Autodesk Inventor part; units mm, degrees
ref_plane "YZ Plane" through (0, 0, 0) normal (1, 0, 0) x (0, 1, 0)
ref_plane "XZ Plane" through (0, 0, 0) normal (0, 1, 0) x (-1, 0, 0)
ref_plane "XY Plane" through (0, 0, 0) normal (0, 0, 1) x (1, 0, 0)
sketch "Sketch1" plane through (0, 0, 0) normal (0, 0, 1) x (1, 0, 0)
  circle A0 centre (0, 91.8009) radius 38.1 construction
  circle A1 centre (0, -91.8009) radius 38.1 construction
  line L0 (0, 91.8009) -> (0, -91.8009) construction
  circle A2 centre (-25.4, 0) radius 57.15 construction
  circle A3 centre (0, 91.8009) radius 14.2875
  circle A4 centre (0, -91.8009) radius 14.2875
  circle A5 centre (0, -91.8009) radius 33.3375 construction
  circle A6 centre (0, 91.8009) radius 33.3375 construction
  circle A7 centre (-142.9967, -39.6875) radius 14.3256 construction
  circle A8 centre (0, -91.8009) radius 23.876 construction
  line L1 (-142.9967, -39.6875) -> (0, -91.8009) construction
  circle A9 centre (-142.9967, 39.6875) radius 14.3256 construction
  circle A10 centre (0, 91.8009) radius 23.876 construction
  line L2 (0, 91.8009) -> (-142.9967, 39.6875) construction
  circle A11 centre (-142.9967, 39.6875) radius 39.6875 construction
  circle A12 centre (-142.9967, -39.6875) radius 39.6875 construction
  line L3 (-142.9967, 39.6875) -> (-142.9967, -39.6875) construction
  line L4 (-138.9458, 25.9466) -> (6.7516, 68.8994) construction
  line L5 (-9.5669, 113.6764) -> (-148.7368, 52.8128) construction
  line L6 (-138.9458, -25.9466) -> (6.7516, -68.8994) construction
  line L7 (-13.5443, -111.4635) -> (-134.8702, -27.89) construction
  circle A13 centre (-142.9967, 39.6875) radius 14.2875
  circle A14 centre (-142.9967, -39.6875) radius 14.2875
  circle A15 centre (-187.9418, -47.625) radius 5.9531 construction
  circle A16 centre (-187.9418, -47.625) radius 9.525
  circle A17 centre (-187.9418, -47.625) radius 17.4625 construction
  circle A18 centre (-187.9418, -47.625) radius 17.4625 construction
  circle A19 centre (-187.9418, -47.625) radius 17.4625 construction
  circle A20 centre (-187.9418, -47.625) radius 17.4625 construction
  circle A21 centre (-187.9418, -47.625) radius 17.4625 construction
  circle A22 centre (-19.05, 0) radius 57.15 construction
  circle A23 centre (-187.9418, -47.625) radius 26.9875
  line L8 (-241.3, 101.6) -> (-215.9, 101.6) construction
  line L9 (-215.9, 101.6) -> (-215.9, -101.6) construction
  line L10 (-215.9, -101.6) -> (-241.3, -101.6) construction
  line L11 (-241.3, -101.6) -> (-241.3, 101.6)
  line L12 (-142.9967, -39.6875) -> (-187.9418, -47.625) construction
  line L13 (-77.6563, 63.5) -> (-77.6563, -63.5) construction
  line L14 (-22.4906, -57.0463) -> (2.007, -58.5239)
  arc A24 (2.007, 58.5239) -> (27.142, 111.1581) centre (0, 91.8009) ccw
  arc A25 (-22.4906, 57.0463) -> (-22.4906, -57.0463) centre (-19.05, 0) ccw
  line L15 (2.007, 58.5239) -> (-22.4906, 57.0463)
  arc A26 (27.142, -111.1581) -> (2.007, -58.5239) centre (0, -91.8009) ccw
  arc A27 (3.8774, 143.7787) -> (-0.8591, 145.6978) centre (0, 141.0134) ccw
  circle A28 centre (0, 91.8009) radius 44.45 construction
  line L16 (3.8774, 143.7787) -> (27.142, 111.1581)
  line L17 (-0.8591, 145.6978) -> (-241.3, 101.6)
  arc A29 (-0.8591, -145.6978) -> (3.8774, -143.7787) centre (0, -141.0134) ccw
  line L18 (-241.3, -101.6) -> (-0.8591, -145.6978)
  line L19 (27.142, -111.1581) -> (3.8774, -143.7787)
  circle A30 centre (0, -91.8009) radius 44.45 construction
  line L20 (0, 112.8194) -> (0, 70.7824) construction
  line L21 (-142.9967, 60.706) -> (-142.9967, 18.669) construction
  line L22 (-142.9967, -18.669) -> (-142.9967, -60.706) construction
  line L23 (0, -70.7824) -> (0, -112.8194) construction
  line L24 (-228.6, 50.8) -> (-228.6, -50.8) construction
  line L25 (-187.9418, -15.875) -> (-187.9418, -79.375) construction
  circle A31 centre (-187.9418, -47.625) radius 17.4625 construction
  point P0 (0, 0)
  point P1 (0, 0)
  point P2 (-172.8189, -38.8937)
  point P3 (-187.9418, -30.1625)
  point P4 (-203.0648, -38.8938)
  point P5 (-203.0648, -56.3563)
  point P6 (-187.9418, -65.0875)
  point P7 (-215.9, 0)
  point P8 (-228.6, 0)
  point P9 (-228.6, 0)
  point P10 (-228.6, 101.6)
  point P11 (-172.8189, -56.3562)
  dimension "d15" = 34.925
  dimension "d0" = 76.2
  dimension "d1" = 76.2
  dimension "d2" = 114.3
  dimension "d4" = 183.6018
  dimension "d5" = 28.575
  dimension "d6" = 19.05
  dimension "d7" = 28.6512
  dimension "d8" = 47.752
  dimension "d9" = 79.375
  dimension "d10" = 142.9967
  dimension "d11" = 152.1968
  dimension "d12" = 28.575
  dimension "d13" = 11.9062
  dimension "d14" = 19.05
  dimension "d18" = 360
  dimension "d20" = 6.35
  dimension "d21" = 53.975
  dimension "d22" = 25.4
  dimension "d23" = 203.2
  dimension "d24" = 241.3
  dimension "d26" = 127
  dimension "d29" = 9.525
  dimension "d30" = 6.35
  dimension "d32" = 42.037
  dimension "d33" = 42.037
  dimension "d34" = 42.037
  dimension "d35" = 42.037
  dimension "d36" = 25.4
  dimension "d44" = 101.6
  dimension "d45" = 53.975
  dimension "d46" = 63.5
extrude "Extrusion1" add sketch "Sketch1" along normal blind 6.35 contours L11 L17 A27 L16 A24 L15 A25 L14 A26 L19 A29 L18
hole "Hole1" at (-172.8189, -38.8937, 0) at (-187.9418, -30.1625, 0) at (-203.0648, -38.8938, 0) at (-203.0648, -56.3563, 0) at (-187.9418, -65.0875, 0) at (-77.6563, 63.5, 0) at (-77.6563, -63.5, 0) at (0, 112.8194, 0) at (0, 70.7824, 0) at (-142.9967, 60.706, 0) at (-142.9967, 18.669, 0) at (-142.9967, -18.669, 0) at (-142.9967, -60.706, 0) at (0, -70.7824, 0) at (0, -112.8194, 0) at (-228.6, 50.8, 0) at (-228.6, 0, 0) at (-228.6, -50.8, 0) at (-187.9418, -79.375, 0) at (-187.9418, -15.875, 0) at (0, -141.0134, 0) at (0, 141.0134, 0) direction (0, 0, 1) diameter 5.1054 end through all
properties part number "GP6-002" material "Polycarbonate, Smoke"
Geometry: final body of the model. Coordinates: model frame, mm. A direction names the side the tool comes from. Give positions to 0.01 mm unless a question says otherwise; leave off trailing zeros. Write each loop counter-clockwise with the first axis right and the second up, starting at its lowest first coordinate (ties: lowest second). Pieces come first, ordered by that corner, then holes. Notation, with made-up numbers: (79, 7) -> (112, 7) arc R7 cw to (112, 15) -> close; hole circle Ø11 at (8, 6.5). An arc over 180 degrees is marked (long way). Answer in a Markdown table with one row per item.
(1) Section query A-A on x = -180. Return loops of the section in (y, z).
Answers below:
| item | result |
|---|---|
| outline | (-112.84, 0) -> (-73.42, 0) -> (-73.42, 6.35) -> (-112.84, 6.35) -> close; (-21.83, 0) -> (112.84, 0) -> (112.84, 6.35) -> (-21.83, 6.35) -> close |
(2) Section query B-B on z = 4. State how many separate pieces and enclosed holes the cut face has, then the cut area to 3 significant figures.
Answers below:
| item | result |
|---|---|
| separate pieces | 1 |
| enclosed holes | 22 |
| area | 51,200 mm^2 |
(3) Section query D-D on x = -19.05. Return loops of the section in (y, z), then the cut area to 3 significant figures.
Answers below:
| item | result |
|---|---|
| outline | (-142.36, 0) -> (-57.25, 0) -> (-57.25, 6.35) -> (-142.36, 6.35) -> close; (57.25, 0) -> (142.36, 0) -> (142.36, 6.35) -> (57.25, 6.35) -> close |
| area | 1,080 mm^2 |
(4) Ray query, line 1 along X through (y, z) = (-29.5, 1.5); line 2 along X through (y, z) = (49, 1.75); line 3 along Y through (x, z) = (-163.5, 5.75). Return the intervals inside material, ascending. Write a range as [from, to].
Answers below:
| item | result |
|---|---|
| line 1 | [-241.3, -207.94], [-167.95, -153.01], [-132.98, -68] |
| line 2 | [-241.3, -230.41], [-226.79, -153.83], [-132.16, -48.46] |
| line 3 | [-115.87, -59.07], [-36.18, 115.87] |
(5) Draft query along X for faces 3 (the flat face through (-122.76, -123.34, 3.13)), 4 (the flat face through (15.7, -127.2, 3.1)), 5 (the cylindrical face through (7.681, 79.754, 3.131)), 6 (the flat face through (-106, 2, 0)). Return one class per face: +X half, -X half, draft (parallel to the pull), parting line (faces both ways), or undercut.
Answers below:
| item | result |
|---|---|
| face 3 | -X half |
| face 4 | +X half |
| face 5 | undercut |
| face 6 | draft |
(6) Set-up query: faces 1 (the flat face through (-10.413, -57.775, 3.131)), 2 (the flat face through (-106, 2, 6.35)). Return all of +Z, -Z, +X, -X, +Y, -Y with unobstructed straight access to the full face (end or side cutting, diameter ignored); none if empty.
Answers below:
| item | result |
|---|---|
| face 1 | +Z, -Z, +X |
| face 2 | +Z, +X, -X, +Y, -Y |
(7) Section query C-C on x = -136.5. Return loops of the section in (y, z).
Answers below:
| item | result |
|---|---|
| outline | (-120.82, 0) -> (-52.41, 0) -> (-52.41, 6.35) -> (-120.82, 6.35) -> close; (-26.96, 0) -> (26.96, 0) -> (26.96, 6.35) -> (-26.96, 6.35) -> close; (52.41, 0) -> (120.82, 0) -> (120.82, 6.35) -> (52.41, 6.35) -> close |
(8) Pin query (flat end, axial travel): pin 1 (4.5 mm diameter, centred on x = -143, y = -60.71, fed in from -Z). Return the tip coordinate at first contact, or that it passes through.
Answers below:
| item | result |
|---|---|
| pin 1 | through |
